The listing builds one solid part. Answer for the finished solid, in the listing's coordinates (mm). Face numbers are marked on the shaded views. A direction names the side the tool comes from. Round coordinates to 2 decimals unless told otherwise and drop trailing zeros. Order: outer loops, then holes, each group sorted by start corner. A loop starts at its lowest first (then second) coordinate and runs counter-clockwise, first axis right, second up. Notation, with made-up numbers: (-33, 13.5) -> (-15, 13.5) arc R22 ccw to (-15, 45.5) -> close; hole circle Ø10 at (-3.75, 69.5). An arc over 180 degrees is marked (long way). Answer in a Markdown table with one row per item. Add a question column.
```python
from build123d import *

# Parameters (mm, degrees)
BOSS_EXTRUDE1_DEPTH = 16.6
SKETCH2_R           = 1.65
CUT_EXTRUDE1_DEPTH  = 17.4
CHAMFER1_SIZE       = 0.4
FILLET1_R           = 1


with BuildPart() as part:
    # Sketch1 → Boss-Extrude1 (new body)
    with BuildSketch(Plane.XY):
        Polygon((0, 0), (8.4, 0), (8.4, 3), (-8, 3), (-8, -15), (0, -15), align=None)
    extrude(amount=BOSS_EXTRUDE1_DEPTH)

    # Sketch2 → Cut-Extrude1 (cut, through all)
    with BuildSketch(Plane.ZY.offset(8)):
        with Locations((3.8, -7.2)):
            Circle(SKETCH2_R)
        with Locations((12.8, -7.2)):
            Circle(SKETCH2_R)
    extrude(amount=-CUT_EXTRUDE1_DEPTH, mode=Mode.SUBTRACT)

    # Chamfer1
    chamfer1_edges = [part.edges().sort_by_distance(p)[0] for p in [
        (-8, 3, 8.3),
        (8.4, 3, 8.3),
        (0.2, 3, 16.6),
        (0.2, 3, 0),
    ]]
    chamfer(chamfer1_edges, length=CHAMFER1_SIZE)

    # Fillet1
    fillet1_edges = [part.edges().sort_by_distance(p)[0] for p in [
        (0, -15, 8.3),
        (-8, -15, 8.3),
        (8.4, 0, 8.3),
    ]]
    fillet(fillet1_edges, radius=FILLET1_R)


solid = part.part
```
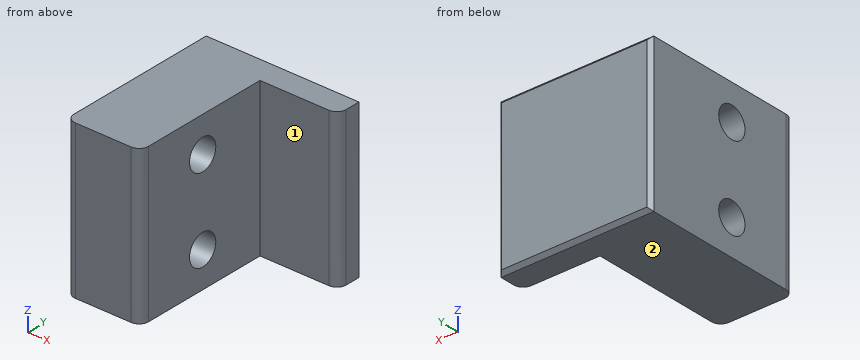
1. The part is cut by section A-A (y = -7.2). Give the vertices of the cut face in (x, z), then the cut area to 3 significant figures.
2. Straight lines are drawn through the part: line 1 along Y through (x, z) = (-3.5, 12.8); line 2 along X through (y, z) = (-0.75, 13.5); line 3 along Y through (x, z) = (3.75, 10.25). For each, find the intervals that lie inside material, in ascending order.
3. The part is cut by section B-B (z = 3.8). Give the vertices of the cut face in (x, y), then the cut area to 3 significant figures.
4. Each of these flat-tipped pins is pushed along its axis until it touches: pin 1 (6 mm diameter, centred on x = 4, y = -10.5, fed in from +Z); pin 2 (5 mm diameter, centred on y = -10.5, z = 14.5, fed in from +X); pin 3 (8 mm diameter, centred on x = 3.5, z = 9, fed in from -Y). Where does it stop, or does it pass through?
5. The part is cut by section C-C (x = 7). Give the vertices of the cut face in (y, z), then the cut area to 3 significant figures.
6. For the marked faces 1 and 2, determine the directions among +Z, -Z, +X, -X, +Y, -Y from which every point of the face is accessible in a straight line to the end or side of a thin tool.
7. The part is cut by section D-D (z = 1). Give the vertices of the cut face in (x, y), then the cut area to 3 significant figures.
Report:
| question | item | result |
|---|---|---|
| 1 | outline | (-8, 0) -> (0, 0) -> (0, 2.15) -> (-8, 2.15) -> close; (-8, 5.45) -> (0, 5.45) -> (0, 11.15) -> (-8, 11.15) -> close; (-8, 14.45) -> (0, 14.45) -> (0, 16.6) -> (-8, 16.6) -> close |
| 1 | area | 80.0 mm^2 |
| 2 | line 1 | y = -15 to -8.85, -5.55 to 3 |
| 2 | line 2 | x = -8 to 0 |
| 2 | line 3 | y = 0 to 3 |
| 3 | outline | (-8, -14) arc R1 ccw to (-7, -15) -> (-1, -15) arc R1 ccw to (0, -14) -> (0, -8.85) -> (-8, -8.85) -> close; (-8, -5.55) -> (0, -5.55) -> (0, 0) -> (7.4, 0) arc R1 ccw to (8.4, 1) -> (8.4, 2.6) -> (8, 3) -> (-7.6, 3) -> (-8, 2.6) -> close |
| 3 | area | 142 mm^2 |
| 4 | pin 1 | passes through |
| 4 | pin 2 | stops at x = 0 |
| 4 | pin 3 | stops at y = -14.87 |
| 5 | outline | (0, 0) -> (2.6, 0) -> (3, 0.4) -> (3, 16.2) -> (2.6, 16.6) -> (0, 16.6) -> close |
| 5 | area | 49.6 mm^2 |
| 6 | face 1 | +Z, -Z, +X, -Y |
| 6 | face 2 | -Z, +X, -X, +Y, -Y |
| 7 | outline | (-8, -14) arc R1 ccw to (-7, -15) -> (-1, -15) arc R1 ccw to (0, -14) -> (0, 0) -> (7.4, 0) arc R1 ccw to (8.4, 1) -> (8.4, 2.6) -> (8, 3) -> (-7.6, 3) -> (-8, 2.6) -> close |
| 7 | area | 168 mm^2 |
